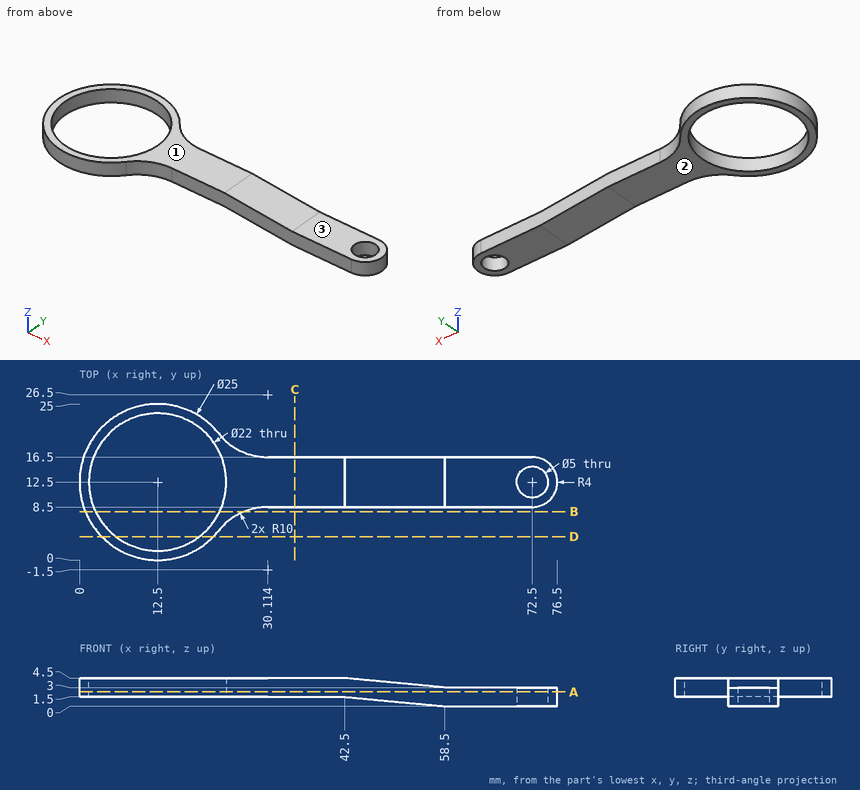
Geometry: see drawing. Coordinates: mm, zero at the bounding-box minimum. A direction names the side the tool comes from. Give positions to 0.01 mm unless a question says otherwise; leave off trailing zeros. Order: outer loops, then holes, each group sorted by start corner. A loop starts at its lowest first (then second) coordinate and runs counter-clockwise, first axis right, second up. Notation, with made-up numbers: (3.25, 41) - (53.25, 41) arc R4 ccw to (53.25, 47) - close; hole circle Ø4 at (42.25, 44.25). An arc over 180 degrees is marked (long way). Write each question's results on one line, items separated by ' | '.
Item 1: Access query for the marked faces 1, 2 and 3. Directions: +Z, -Z, +X, -X, +Y, -Y. A direction counts if a zero-diameter tool reaches every point of the face in a straight line with its end or side. Return the directions, or none.
A:
face 1: +Z, +X, -X, +Y, -Y | face 2: -Z, -X, +Y, -Y | face 3: +Z, +X, +Y, -Y
Item 2: Section C-C (x = 34.5). Return loops of the section in (y, z), and give its area (3 significant figures).
A:
outline: (8.5, 1.5) - (16.5, 1.5) - (16.5, 4.5) - (8.5, 4.5) - close | area: 24.0 mm^2
Item 3: Section B-B (y = 7.75). Return loops of the section in (x, z).
A:
outline: (0.94, 1.5) - (2.58, 1.5) - (2.58, 4.5) - (0.94, 4.5) - close; (22.42, 1.5) - (26.31, 1.5) - (26.31, 4.5) - (22.42, 4.5) - close
Item 4: Material intervals for line 1 along Y through (x, z) = (12, 3.45); line 2 along X through (y, z) = (13, 2.15); line 3 along Z through (x, y) = (61, 11.5), sorted ascending.
A:
line 1: y = 0.01 to 1.51, 23.49 to 24.99 | line 2: x = 0.01 to 1.51, 23.49 to 70.05, 74.95 to 76.47 | line 3: z = 0 to 3
Item 5: Contact query for flat-ended pins moving along their axis: pin 1 Ø3 at (x, y) = (72.5, 12.5) entering from -Z; pin 2 Ø2 at (x, z) = (17, 2) entering from -Y; pin 3 Ø1 at (x, z) = (41.5, 2.5) entering from -Y; pin 4 Ø12 at (x, y) = (53, 12.5) entering from +Z. Output: stop coordinate, or through.
A:
pin 1: passes through | pin 2: stops at y = 0.5 | pin 3: stops at y = 8.5 | pin 4: stops at z = 4.08
Item 6: Section A-A (z = 2.3). Return loops of the section in (x, y).
A:
outline: (22.29, 4.72) arc R10 cw to (30.11, 8.5) - (72.5, 8.5) arc R4 ccw to (72.5, 16.5) - (30.11, 16.5) arc R10 cw to (22.29, 20.28) arc R12.5 ccw (long way) to start; hole circle Ø22 at (12.5, 12.5); hole circle Ø5 at (72.5, 12.5)
Item 7: Section D-D (y = 3.75). Return loops of the section in (x, z).
A:
outline: (3.57, 1.5) - (5.83, 1.5) - (5.83, 4.5) - (3.57, 4.5) - close; (19.17, 1.5) - (21.43, 1.5) - (21.43, 4.5) - (19.17, 4.5) - close
